Geometry: final body of the model. Coordinates: model frame, mm. Face numbers are marked on the shaded views. Round coordinates to 2 decimals unless told otherwise and drop trailing zeros. Answer as a JSON object with one key per item and string values. Group by question number.
Item 1: Section A-A (y = 8). Count the separate pieces of the cut face and the enclosed holes in it, plus the area to 3 significant figures.
Item 2: First-contact query: pin 1 (3 mm diameter, centred on x = 11.5, y = 9, fed in from +Z); pin 2 (1.6 mm diameter, centred on y = -0.5, z = 0.5, fed in from +X); pin 3 (1.1 mm diameter, centred on x = -13.5, z = 3, fed in from +Y). Flat tips, straight axial feed; report the tip coordinate or a pass-through.
Item 3: Line query: line 1 (X direction, y = -12.5, z = 3.55); line 2 (Y direction, x = -8, z = 0.9) (3 decimals); line 3 (Y direction, x = 8, z = 0.7) (1 decimal). Output: solid intervals per line, ascending.
Item 4: Draft query along Y for the marked faces 1 and 2. Return one class per face: released by +Y, released by -Y, zero draft, split by the parting line, or undercut.
```python
from build123d import *

# Parameters (mm, degrees)
SKETCH1_W           = 32
SKETCH1_H           = 62
BOSS_EXTRUDE4_DEPTH = 2
SKETCH6_W           = 28
SKETCH6_H           = 2
SKETCH6_W_2         = 7
SKETCH6_H_2         = 1
SKETCH6_W_3         = 1
SKETCH6_H_3         = 30
BOSS_EXTRUDE6_DEPTH = 2
SKETCH7_R           = 6
SKETCH7_R_2         = 5.000319164
CUT_EXTRUDE3_DEPTH  = 1.5
SKETCH8_W           = 2
SKETCH8_H           = 38
CUT_EXTRUDE5_DEPTH  = 2
SKETCH26_W          = 10.2
SKETCH26_H          = 2
CUT_EXTRUDE11_DEPTH = 2
FILLET3_R           = 1
FILLET5_R           = 4
FILLET6_R           = 1


with BuildPart() as part:
    # Sketch1 → Boss-Extrude4 (new body)
    with BuildSketch(Plane.XY):
        Rectangle(SKETCH1_W, SKETCH1_H)
    extrude(amount=BOSS_EXTRUDE4_DEPTH)

    # Sketch6 → Boss-Extrude6 (add)
    with BuildSketch(Plane.XY.offset(2)):
        with Locations((0, 27)):
            Rectangle(SKETCH6_W, SKETCH6_H)
        with Locations((-8.6, -28.5)):
            Rectangle(SKETCH6_W_2, SKETCH6_H_2)
        with Locations((-13.5, -11)):
            Rectangle(SKETCH6_W_3, SKETCH6_H_3)
        with Locations((13.5, -11)):
            Rectangle(SKETCH6_W_3, SKETCH6_H_3)
        with Locations((8.6, -28.5)):
            Rectangle(SKETCH6_W_2, SKETCH6_H_2)
    extrude(amount=BOSS_EXTRUDE6_DEPTH)

    # Sketch7 → Cut-Extrude3 (cut)
    # profile 1 of 4: a face of its own
    with BuildSketch(Plane(origin=(0, 0, 0), x_dir=(-1, 0, 0), z_dir=(0, 0, -1))):
        with Locations((8, 23)):
            Circle(SKETCH7_R)
        with Locations((8, 23)):
            Circle(SKETCH7_R_2, mode=Mode.SUBTRACT)
    # profile 2 of 4: a face of its own
    with BuildSketch(Plane(origin=(0, 0, 0), x_dir=(-1, 0, 0), z_dir=(0, 0, -1))):
        with Locations(Location((-8, 23, 0), (0, 0, 180))):
            Circle(SKETCH7_R)
        with Locations(Location((-8, 23, 0), (0, 0, 180))):
            Circle(SKETCH7_R_2, mode=Mode.SUBTRACT)
    # profile 3 of 4: a face of its own
    with BuildSketch(Plane(origin=(0, 0, 0), x_dir=(-1, 0, 0), z_dir=(0, 0, -1))):
        Polygon((7.449564134, 19.902085928), (7.449564134, 26.125), (8.241594022, 26.125), (8.241594022, 20.615660025), (9.067247821, 20.615660025), (9.067247821, 19.902085928), align=None)
    # profile 4 of 4: a face of its own
    with BuildSketch(Plane(origin=(0, 0, 0), x_dir=(-1, 0, 0), z_dir=(0, 0, -1))):
        with BuildLine():
            Line((-7.146948941, 25.376463263), (-10.108343711, 25.376463263))
            Line((-10.108343711, 25.376463263), (-10.108343711, 26.031506849))
            Line((-10.108343711, 26.031506849), (-5.96886675, 26.031506849))
            Line((-5.96886675, 26.031506849), (-5.96886675, 25.471108344))
            add(Edge.make_bspline(
                [(-5.96886675, 25.471108344), (-6.141971745, 25.332246025), (-6.393074253, 25.128048459), (-6.717159934, 24.860884743), (-6.938355226, 24.675665503), (-7.14521645, 24.500220273), (-7.337036334, 24.334147369), (-7.515021507, 24.179302523), (-7.729935684, 23.986290529), (-7.97797696, 23.749213926), (-8.254030773, 23.459208844), (-8.501907476, 23.159401339), (-8.692650042, 22.906276826), (-8.827236908, 22.7005165), (-8.914850872, 22.548009682), (-8.987343685, 22.394896597), (-9.047188475, 22.243011314), (-9.09511833, 22.092158743), (-9.14011918, 21.893098726), (-9.153639256, 21.741878323), (-9.153175592, 21.641718555)],
                knots=[0, 0, 0, 0, 0.130040941, 0.189652936, 0.246118775, 0.299098592, 0.348595518, 0.394796265, 0.437339888, 0.517855819, 0.595805403, 0.671798956, 0.745699159, 0.781390574, 0.815816171, 0.848675559, 0.880566293, 0.911416805, 0.941336485, 1, 1, 1, 1], degree=3))
            add(Edge.make_bspline(
                [(-9.153175592, 21.641718555), (-9.155082227, 21.552888892), (-9.144519697, 21.423140421), (-9.117017207, 21.256160493), (-9.086176124, 21.141966589), (-9.049844313, 21.034116343), (-9.002140941, 20.934767093), (-8.946696453, 20.842593454), (-8.883433554, 20.757430331), (-8.810058845, 20.68075797), (-8.724921804, 20.615898841), (-8.631522153, 20.558997899), (-8.52626692, 20.514689776), (-8.41184588, 20.478122069), (-8.238594227, 20.444792793), (-8.102433508, 20.436059356), (-8.00871731, 20.436239103)],
                knots=[0, 0, 0, 0, 0.139728186, 0.204784982, 0.266341208, 0.325916068, 0.383845258, 0.439595464, 0.495191981, 0.550699936, 0.606173196, 0.663381541, 0.722556505, 0.785650329, 0.852353324, 1, 1, 1, 1], degree=3))
            add(Edge.make_bspline(
                [(-8.00871731, 20.436239103), (-7.916381499, 20.437963905), (-7.780275222, 20.44531508), (-7.607573636, 20.484711085), (-7.489539865, 20.524886263), (-7.37894443, 20.575440972), (-7.278056027, 20.640240509), (-7.183251352, 20.713479274), (-7.098817495, 20.800136263), (-7.023700984, 20.896089204), (-6.955094248, 20.998590264), (-6.898475794, 21.110250127), (-6.849345945, 21.228689465), (-6.811085908, 21.35564304), (-6.77026818, 21.538429964), (-6.756832641, 21.68156666), (-6.752179328, 21.778704857)],
                knots=[0, 0, 0, 0, 0.134196199, 0.196562655, 0.256347301, 0.314798293, 0.372427992, 0.429881299, 0.488208125, 0.547352693, 0.606466609, 0.666785475, 0.728614883, 0.792224418, 0.858834798, 1, 1, 1, 1], degree=3))
            Line((-6.752179328, 21.778704857), (-5.99377335, 21.778704857))
            add(Edge.make_bspline(
                [(-5.99377335, 21.778704857), (-5.997486049, 21.626043992), (-6.022968038, 21.403553268), (-6.087771701, 21.119090113), (-6.154533355, 20.925565149), (-6.235258471, 20.744918428), (-6.332722054, 20.577794308), (-6.448082734, 20.425562017), (-6.577838607, 20.287424291), (-6.719500697, 20.163361209), (-6.874023412, 20.058172324), (-7.036357792, 19.965442189), (-7.21032699, 19.892804952), (-7.393628445, 19.834880004), (-7.656331886, 19.77911898), (-7.861386403, 19.766430592), (-8, 19.765006227)],
                knots=[0, 0, 0, 0, 0.143256095, 0.209727491, 0.273583639, 0.335170915, 0.395274724, 0.454838861, 0.51413324, 0.572990339, 0.631272766, 0.689392012, 0.748255565, 0.807926753, 0.869702493, 1, 1, 1, 1], degree=3))
            add(Edge.make_bspline(
                [(-8, 19.765006227), (-8.141000178, 19.763539171), (-8.347034063, 19.780521722), (-8.612322806, 19.829086312), (-8.79374631, 19.885647608), (-8.96555498, 19.953126433), (-9.125345548, 20.038241229), (-9.273376818, 20.138643722), (-9.409243356, 20.253208897), (-9.531806427, 20.381382972), (-9.637390513, 20.522817866), (-9.728706814, 20.67446601), (-9.80046805, 20.839449985), (-9.857663027, 21.014979064), (-9.914464012, 21.270428027), (-9.92596825, 21.470796687), (-9.927770859, 21.606849315)],
                knots=[0, 0, 0, 0, 0.139977399, 0.205129271, 0.267661615, 0.328584124, 0.388397961, 0.44723, 0.506092426, 0.564763589, 0.623116047, 0.681221368, 0.740343609, 0.801549192, 0.864527945, 1, 1, 1, 1], degree=3))
            add(Edge.make_bspline(
                [(-9.927770859, 21.606849315), (-9.928242812, 21.72559986), (-9.915013433, 21.903984583), (-9.870131257, 22.138500082), (-9.822350184, 22.313101458), (-9.762269632, 22.486490626), (-9.690286657, 22.659318649), (-9.602323879, 22.829621189), (-9.469377828, 23.054284468), (-9.285596836, 23.323787524), (-9.052240665, 23.632715958), (-8.802279105, 23.919912782), (-8.579780596, 24.144048337), (-8.391224564, 24.317762692), (-8.241857572, 24.454065056), (-8.081858709, 24.594549679), (-7.913468988, 24.741333436), (-7.734490681, 24.891808295), (-7.479898932, 25.106191886), (-7.283114849, 25.268511143), (-7.146948941, 25.376463263)],
                knots=[0, 0, 0, 0, 0.073605163, 0.110554154, 0.147890148, 0.185738035, 0.22426503, 0.263861232, 0.3044708, 0.386061806, 0.465952502, 0.544398616, 0.621927399, 0.661628021, 0.703351885, 0.747296454, 0.793637954, 0.841849967, 0.892268874, 1, 1, 1, 1], degree=3))
        make_face()
    extrude(amount=-CUT_EXTRUDE3_DEPTH, mode=Mode.SUBTRACT)

    # Sketch8 → Cut-Extrude5 (cut)
    with BuildSketch(Plane(origin=(0, 0, 0), x_dir=(-1, 0, 0), z_dir=(0, 0, -1))):
        with Locations((6, -7)):
            Rectangle(SKETCH8_W, SKETCH8_H)
        with Locations((2, -7)):
            Rectangle(SKETCH8_W, SKETCH8_H)
        with Locations((-2, -7)):
            Rectangle(SKETCH8_W, SKETCH8_H)
        with Locations((-6, -7)):
            Rectangle(SKETCH8_W, SKETCH8_H)
        with Locations((-10, -7)):
            Rectangle(SKETCH8_W, SKETCH8_H)
        with Locations((10, -7)):
            Rectangle(SKETCH8_W, SKETCH8_H)
    extrude(amount=-CUT_EXTRUDE5_DEPTH, mode=Mode.SUBTRACT)

    # Sketch26 → Cut-Extrude11 (cut)
    with BuildSketch(Plane.XZ.offset(31)):
        with Locations((0, 1)):
            Rectangle(SKETCH26_W, SKETCH26_H)
    extrude(amount=-CUT_EXTRUDE11_DEPTH, mode=Mode.SUBTRACT)

    # Fillet3
    fillet3_edges = [part.edges().sort_by_distance(p)[0] for p in [
        (-9, 12, 1),
        (-5, 12, 1),
        (-1, 12, 1),
        (3, 12, 1),
        (7, 12, 1),
        (11, 12, 1),
        (9, 12, 1),
        (5, 12, 1),
        (1, 12, 1),
        (-3, 12, 1),
        (-7, 12, 1),
        (-11, 12, 1),
        (-5, -26, 1),
        (-1, -26, 1),
        (3, -26, 1),
        (7, -26, 1),
        (11, -26, 1),
        (9, -26, 1),
        (5, -26, 1),
        (1, -26, 1),
        (-3, -26, 1),
        (-7, -26, 1),
        (-9, -26, 1),
        (-11, -26, 1),
    ]]
    fillet(fillet3_edges, radius=FILLET3_R - 0.0001)  # a hair under: the kernel refuses the full size

    # Fillet5
    fillet5_edges = [part.edges().sort_by_distance(p)[0] for p in [
        (16, -31, 1),
        (-16, -31, 1),
        (-16, 31, 1),
        (16, 31, 1),
    ]]
    fillet(fillet5_edges, radius=FILLET5_R)

    # Fillet6
    fillet6_edges = [part.edges().sort_by_distance(p)[0] for p in [
        (8.55, -31, 0),
        (-5.1, -30, 0),
        (0, -29, 0),
        (5.1, -30, 0),
        (-16, 0, 0),
        (-8.55, -31, 0),
        (0, 31, 0),
        (16, 0, 0),
        (14.828427125, 29.828427125, 0),
        (14.828427125, -29.828427125, 0),
        (-14.828427125, -29.828427125, 0),
        (-14.828427125, 29.828427125, 0),
    ]]
    fillet(fillet6_edges, radius=FILLET6_R)


solid = part.part
```
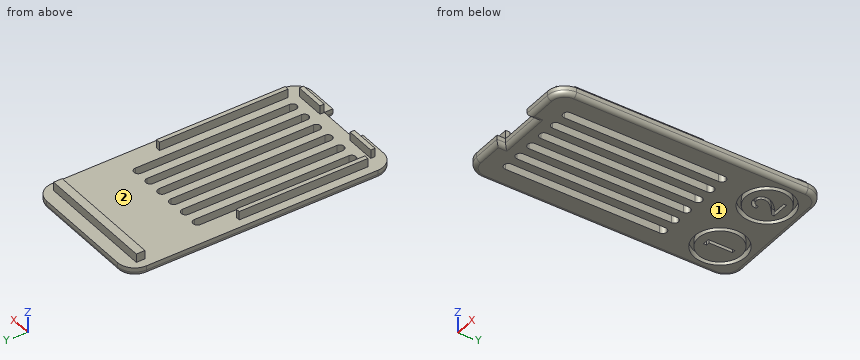
Values:
{
 "1": {"separate pieces": "7", "enclosed holes": "0", "area": "39.6 mm^2"},
 "2": {"pin 1": "stops at z = 2", "pin 2": "stops at x = 16", "pin 3": "stops at y = 28"},
 "3": {"line 1": "x = -14 to -13, 13 to 14", "line 2": "y = -30.995 to 17, 18 to 19.902, 26.125 to 28, 29 to 30.995", "line 3": "y = -31 to 17, 18 to 19.8, 20.4 to 23.7, 24.7 to 25.4, 26 to 28, 29 to 31"},
 "4": {"face 1": "zero draft", "face 2": "undercut"}
}
